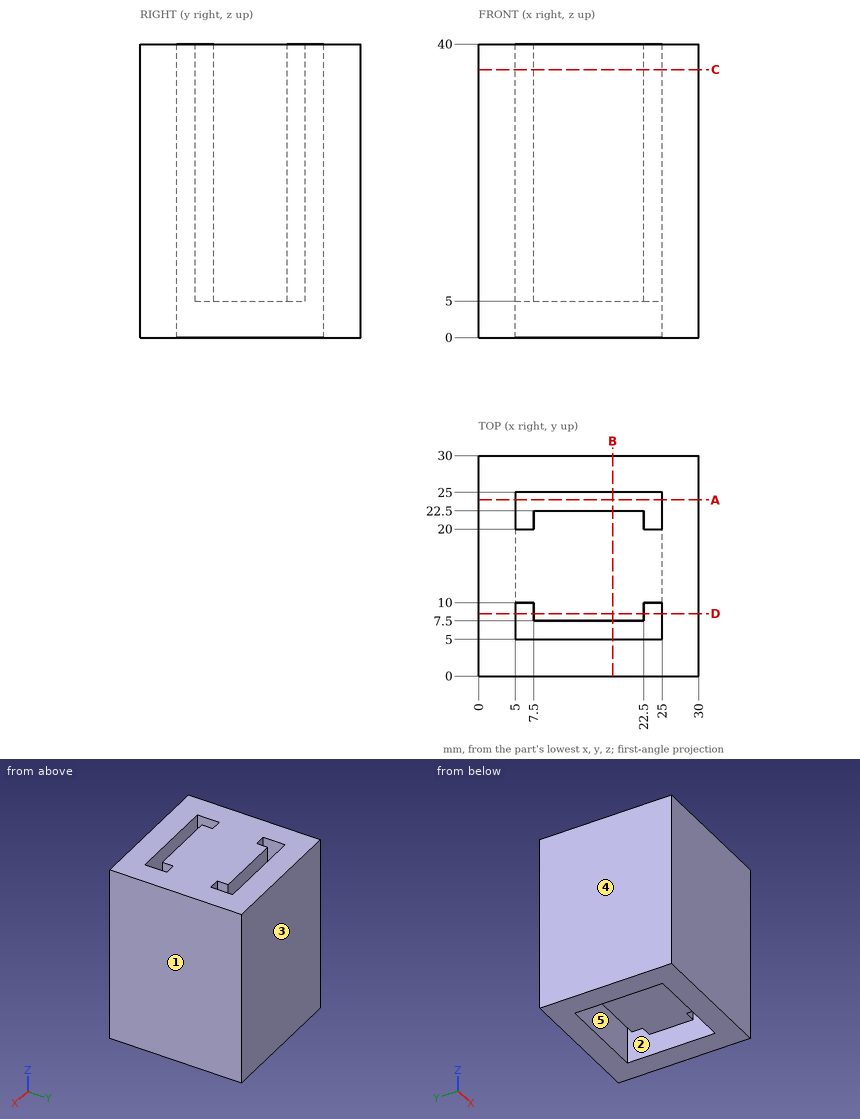
Geometry check sheet. Reference: drawing and pictorial views, mm from the part's lowest x, y, z. A direction names the side the tool comes from. Round coordinates to 2 decimals unless told otherwise and drop trailing zeros. Order: outer loops, then holes, each group sorted by start corner. A loop starts at its lowest first (then second) coordinate and runs counter-clockwise, first axis right, second up. Notation, with made-up numbers: M 8.25,34 L 45.25,34 A32 ccw 45.25,67 Z; hole C -28,76.25 d1. An arc over 180 degrees is marked long. Write item = value, one per line.
Q1. Section check C-C (z = 36.5). Enter the section's corners in (x, y), plus the area to 3 significant figures.
Answer block:
outline = M 0,0 L 30,0 L 30,30 L 0,30 Z; hole M 5,5 L 25,5 L 25,10 L 22.5,10 L 22.5,7.5 L 7.5,7.5 L 7.5,10 L 5,10 Z; hole M 5,20 L 7.5,20 L 7.5,22.5 L 22.5,22.5 L 22.5,20 L 25,20 L 25,25 L 5,25 Z
area = 775 mm^2
Q2. Section check B-B (x = 18.25). Enter the section's corners in (y, z), plus the area to 3 significant figures.
Answer block:
outline = M 0,0 L 5,0 L 5,40 L 0,40 Z; M 7.5,5 L 22.5,5 L 22.5,40 L 7.5,40 Z; M 25,0 L 30,0 L 30,40 L 25,40 Z
area = 925 mm^2
Q3. Release check for a two-part mould opening along X. For the marked faces 3, 4 and 5 record: released by +X, released by -X, zero draft, split by the parting line, or undercut.
Answer block:
face_3 = zero draft
face_4 = released by -X
face_5 = undercut
Q4. Depth check by flat-ended pin: pin 1 Ø1 at (x, y) = (19, 19.5) entering from -Z. Enter the tip coordinate at first touch or a pass-through.
Answer block:
pin_1 = 5
Q5. Scan lines: line 1 (Y direction, x = 16.75, z = 38); line 2 (X direction, y = 9.5, z = 2); line 3 (Y direction, x = 6.25, z = 37). Record each from-to range of solid material in increasing order.
Answer block:
line_1 = 0 to 5, 7.5 to 22.5, 25 to 30
line_2 = 0 to 5, 25 to 30
line_3 = 0 to 5, 10 to 20, 25 to 30
Q6. Section check A-A (y = 24). Enter the section's corners in (x, z).
Answer block:
outline = M 0,0 L 5,0 L 5,40 L 0,40 Z; M 25,0 L 30,0 L 30,40 L 25,40 Z
Q7. Set-up check for the marked faces 1 and 2: record each of +Z, -Z, +X, -X, +Y, -Y from which the full face is reachable in a straight line by a thin tool's end or side.
Answer block:
face_1 = +Z, -Z, +X, +Y, -Y
face_2 = -Z
